Design review of the part built by this model. Coordinates are the model's own, in mm. A direction names the side the tool comes from. Coordinates: 2 decimals unless noted, no trailing zeros. Write each loop counter-clockwise with the first axis right and the second up, starting at its lowest first coordinate (ties: lowest second). Pieces come first, ordered by that corner, then holes.
Q1. Take a section at D-D (x = 33.5). Give the boundary of the cut face in (y, z).
Q2. Take a section at C-C (y = 5). Give the boundary of the cut face in (x, z), and give its area (3 significant figures).
Q3. Machinability: for faces 5 (the flat face through (37.5, 37, 0)), 6 (the flat face through (33, 0, 6)), 7 (the flat face through (0, 35, 0)), 8 (the cylindrical face through (-5, -22, 0)), which of the approach directions +Z, -Z, +X, -X, +Y, -Y give a long, thin tool a straight path to every point of the face, cutting with its end or side? Answer none if there is none.
Q4. Mouldability with a two-part tool opening along X and no side actions: class faces 1 (the flat face through (29.5, 37, 0)), 2 (the flat face through (17, 0, -5)), 3 (the flat face through (0, 0, 10)), 4 (the flat face through (17, 0, 5)) as pulls with the +X half, pulls with the -X half, needs draft (parallel to the pull), parting line crosses it, or undercut.
Q5. Take a section at B-B (x = -5). Give the boundary of the cut face in (y, z).
Q6. Insertion check: pin 1 (8 mm diameter, centred on x = 14.5, y = 25.5, fed in from +Z); pin 2 (6 mm diameter, centred on x = 33, y = -9.5, fed in from +Z); pin 3 (8 mm diameter, centred on y = -26.5, z = -0.5, fed in from -X); pin 4 (5 mm diameter, centred on x = 5.5, z = 6.5, fed in from +Y). Each pin has a flat end and moves straight along its axis. Give the tip position at first contact, or say it passes through.
Q7. Take a section at A-A (y = 27). Give the boundary of the cut face in (x, z).
Q8. For probe 1 along X at (y, z) = (-31, 0); probe 2 along Z at (x, y) = (-5.8, 27); probe 3 along X at (y, z) = (20.5, -2.5), list the stretches that pass through material, from the lowest coordinate up.
```python
from build123d import *

# Parameters (mm, degrees)
SKETCH1_W           = 15
SKETCH1_H           = 70
BOSS_EXTRUDE1_DEPTH = 10
SKETCH2_W           = 20
SKETCH2_H           = 40
BOSS_EXTRUDE2_DEPTH = 5
SKETCH5_W           = 12
SKETCH5_H           = 70
BOSS_EXTRUDE4_DEPTH = 6
SKETCH6_W           = 8
SKETCH6_H           = 8
BOSS_EXTRUDE5_DEPTH = 5
SKETCH7_R           = 4
BOSS_EXTRUDE6_DEPTH = 5
SKETCH8_R           = 5
CUT_EXTRUDE1_DEPTH  = 5


with BuildPart() as part:
    # Sketch1 → Boss-Extrude1 (new, symmetric)
    with BuildSketch(Plane.XY):
        Rectangle(SKETCH1_W, SKETCH1_H)
    extrude(amount=BOSS_EXTRUDE1_DEPTH, both=True)

    # Sketch2 → Boss-Extrude2 (add, symmetric)
    with BuildSketch(Plane.XY):
        with Locations((17.5, 0)):
            Rectangle(SKETCH2_W, SKETCH2_H)
    extrude(amount=BOSS_EXTRUDE2_DEPTH, both=True)

    # Sketch5 → Boss-Extrude4 (add, symmetric)
    with BuildSketch(Plane.XY):
        with Locations((33.5, 0)):
            Rectangle(SKETCH5_W, SKETCH5_H)
    extrude(amount=BOSS_EXTRUDE4_DEPTH, both=True)

    # Sketch6 → Boss-Extrude5 (add)
    with BuildSketch(Plane(origin=(0, 35, 0), x_dir=(1, 0, 0), z_dir=(0, 1, 0))):
        with Locations((33.5, 0)):
            Rectangle(SKETCH6_W, SKETCH6_H)
    extrude(amount=BOSS_EXTRUDE5_DEPTH)

    # Sketch7 → Boss-Extrude6 (add)
    with BuildSketch(Plane.XZ.offset(35)):
        with Locations(Location((33.5, 0, 0), (0, 0, 270))):
            Circle(SKETCH7_R)
    extrude(amount=BOSS_EXTRUDE6_DEPTH)

    # Sketch8 → Cut-Extrude1 (cut)
    with BuildSketch(Plane.ZY.offset(7.5)):
        with Locations(Location((0, 27, 0), (0, 0, 270))):
            Circle(SKETCH8_R)
        with Locations(Location((0, 9, 0), (0, 0, 270))):
            Circle(SKETCH8_R)
        with Locations(Location((0, -9, 0), (0, 0, 270))):
            Circle(SKETCH8_R)
        with Locations(Location((0, -27, 0), (0, 0, 270))):
            Circle(SKETCH8_R)
    extrude(amount=-CUT_EXTRUDE1_DEPTH, mode=Mode.SUBTRACT)


solid = part.part
```
Response:
1. outline: (-40, -4) - (-35, -4) - (-35, -6) - (35, -6) - (35, -4) - (40, -4) - (40, 4) - (35, 4) - (35, 6) - (-35, 6) - (-35, 4) - (-40, 4) - close
2. outline: (-7.5, -10) - (7.5, -10) - (7.5, -5) - (27.5, -5) - (27.5, -6) - (39.5, -6) - (39.5, 6) - (27.5, 6) - (27.5, 5) - (7.5, 5) - (7.5, 10) - (-7.5, 10) - (-7.5, 3) - (-2.5, 3) - (-2.5, -3) - (-7.5, -3) - close
2. area: 614 mm2
3. face 5: +Z, -Z, +X, +Y
3. face 6: +Z, +X, +Y, -Y
3. face 7: +Z, -Z, -X, +Y
3. face 8: -X
4. face 1: pulls with the -X half
4. face 2: undercut
4. face 3: needs draft
4. face 4: undercut
5. outline: (-35, -10) - (35, -10) - (35, 10) - (-35, 10) - close; hole circle Ø10 at (-27, 0); hole circle Ø10 at (-9, 0); hole circle Ø10 at (9, 0); hole circle Ø10 at (27, 0)
6. pin 1: passes through
6. pin 2: stops at z = 6
6. pin 3: stops at x = -2.5
6. pin 4: stops at y = 35
7. outline: (-7.5, -10) - (7.5, -10) - (7.5, 10) - (-7.5, 10) - (-7.5, 5) - (-2.5, 5) - (-2.5, -5) - (-7.5, -5) - close; (27.5, -6) - (39.5, -6) - (39.5, 6) - (27.5, 6) - close
8. probe 1: x = -2.5 to 7.5, 27.5 to 39.5
8. probe 2: z = -10 to -5, 5 to 10
8. probe 3: x = -7.5 to 7.5, 27.5 to 39.5
